Here's how the part is built. I have some questions about the finished solid (model axes, mm). A direction names the side the tool comes from. Coordinates: 2 decimals unless noted, no trailing zeros. Write each loop counter-clockwise with the first axis right and the second up, starting at its lowest first coordinate (ties: lowest second). Pieces come first, ordered by that corner, then holes. Notation, with made-up numbers: (60, -34) - (66, -34) arc R20 ccw to (66, -23) - close; hole circle Ø10 at (-31.5, 8). An arc over 180 degrees is marked (long way). Answer in a Markdown table with one row per item. Add a question column.
Item 1: If I drill on probe 1 along X at (y, z) = (26, -20.5); probe 2 along Z at (x, y) = (-39, 25.5), over which ranges is the centre line in solid material (lowest first)? Write a range as from..to.
Item 2: We'd pull the mould along Z, two halves only. Please class faces 1 (the face through (-7, 0, -10)), 2 (the face through (6.35, 24, 4)), 3 (the face through (0, 25, -36.512)), 4 (the face through (-1, 26, 44.45)): +Z half, -Z half, draft (parallel to the pull), parting line (faces both ways), or undercut.
Item 3: Imagine slicing it at D-D (z = 0). Please give me the cut outline in (x, y).
Item 4: Imagine slicing it at A-A (y = 32). State how many separate pieces and enclosed holes the cut face has, plus the area to 3 significant figures.
Item 5: Which directions (+Z, -Z, +X, -X, +Y, -Y) give clear straight access to the entire face, cutting with the end or side of a thin tool? Please do faces 5 (the face through (0, 12.7, 40)), 6 (the face through (7.938, 24, 4)), 7 (the face through (-44.45, 25, 1)).
Item 6: I'm going to push flat-ended pins straight in: pin 1 (1.5 mm diameter, centred on x = -4, z = 3, fed in from -Y); pin 2 (4 mm diameter, centred on x = -1.5, z = 23, fed in from -Y). Where does each tip first touch, or does it pass through?
from build123d import *

# Parameters (mm, degrees)
SKETCH1_W           = 88.9
SKETCH1_H           = 88.9
BOSS_EXTRUDE1_DEPTH = 50.8
SHELL1_T            = -1.5875
SKETCH4_R           = 4.7625
CUT_EXTRUDE3_DEPTH  = 51.8
SKETCH5_W           = 15.875
SKETCH5_H           = 73.025
SKETCH5_W_2         = 12.7
SKETCH5_H_2         = 69.85
EXTRUDE_THIN1_DEPTH = 49.2125
SKETCH10_R          = 7.9375
SKETCH10_R_2        = 4.7625
BOSS_EXTRUDE5_DEPTH = 6.35
SKETCH14_W          = 15.875
SKETCH14_H          = 14.2875
BOSS_EXTRUDE7_DEPTH = 7.9375
CUT_EXTRUDE6_START  = -9.525
SKETCH15_W          = 12.7
SKETCH15_H          = 12.7
CUT_EXTRUDE6_DEPTH  = 9.525


with BuildPart() as part:
    # Sketch1 → Boss-Extrude1 (new body)
    with BuildSketch(Plane(origin=(0, 0, 0), x_dir=(1, 0, 0), z_dir=(0, 1, 0))):
        Rectangle(SKETCH1_W, SKETCH1_H)
    extrude(amount=BOSS_EXTRUDE1_DEPTH)

    # Shell1
    shell1_openings = [part.faces().sort_by_distance(p)[0] for p in [
        (0, 0, 0),
    ]]
    offset(amount=SHELL1_T, openings=shell1_openings, kind=Kind.INTERSECTION)

    # Sketch4 → Cut-Extrude3 (cut, through all)
    with BuildSketch(Plane(origin=(0, 50.8, 0), x_dir=(1, 0, 0), z_dir=(0, 1, 0))):
        Circle(SKETCH4_R)
    extrude(amount=-CUT_EXTRUDE3_DEPTH, mode=Mode.SUBTRACT)

    # Sketch5 → Extrude-Thin1 (add)
    with BuildSketch(Plane.XZ.offset(-49.2125)):
        Rectangle(SKETCH5_W, SKETCH5_H)
        Rectangle(SKETCH5_W_2, SKETCH5_H_2, mode=Mode.SUBTRACT)
    extrude(amount=EXTRUDE_THIN1_DEPTH)

    # Sketch10 → Boss-Extrude5 (add)
    with BuildSketch(Plane.XZ.offset(-49.2125)):
        Circle(SKETCH10_R)
        Circle(SKETCH10_R_2, mode=Mode.SUBTRACT)
    extrude(amount=BOSS_EXTRUDE5_DEPTH)

    # Sketch14 → Boss-Extrude7 (add)
    with BuildSketch(Plane.XY.offset(44.45)):
        with Locations((0, 7.14375)):
            Rectangle(SKETCH14_W, SKETCH14_H)
    extrude(amount=-BOSS_EXTRUDE7_DEPTH)

    # Sketch15 → Cut-Extrude6 (cut)
    with BuildSketch(Plane.XY.offset(44.45).offset(CUT_EXTRUDE6_START)):
        with Locations((0, 6.35)):
            Rectangle(SKETCH15_W, SKETCH15_H)
    extrude(amount=CUT_EXTRUDE6_DEPTH, mode=Mode.SUBTRACT)


solid = part.part
Here are the results:
| question | item | result |
|---|---|---|
| 1 | probe 1 | x = -44.45..-42.86, -7.94..-6.35, 6.35..7.94, 42.86..44.45 |
| 1 | probe 2 | z = -44.45..-42.86, 42.86..44.45 |
| 2 | face 1 | draft |
| 2 | face 2 | undercut |
| 2 | face 3 | undercut |
| 2 | face 4 | +Z half |
| 3 | outline | (-44.45, 0) - (-42.86, 0) - (-42.86, 49.21) - (-7.94, 49.21) - (-7.94, 0) - (-6.35, 0) - (-6.35, 42.86) - (-4.76, 42.86) - (-4.76, 50.8) - (-44.45, 50.8) - close; (4.76, 42.86) - (6.35, 42.86) - (6.35, 0) - (7.94, 0) - (7.94, 49.21) - (42.86, 49.21) - (42.86, 0) - (44.45, 0) - (44.45, 50.8) - (4.76, 50.8) - close |
| 4 | separate pieces | 2 |
| 4 | enclosed holes | 2 |
| 4 | area | 827 mm2 |
| 5 | face 5 | +Z, -Y |
| 5 | face 6 | -Y |
| 5 | face 7 | +Z, -Z, -X, +Y, -Y |
| 6 | pin 1 | stops at y = 42.86 |
| 6 | pin 2 | stops at y = 49.21 |
